Here's how the part is built. I have some questions about the finished solid (model axes, mm). Face numbers are marked on the shaded views. A direction names the side the tool comes from. Coordinates: 2 decimals unless noted, no trailing zeros. Write each loop counter-clockwise with the first axis right and the second up, starting at its lowest first coordinate (ties: lowest second). Pieces come first, ordered by that corner, then holes. Notation, with made-up numbers: (23.5, -39.75) -> (74.5, -39.75) arc R24 cw to (74.5, -8.75) -> close; hole circle Ø8 at (-9.75, -10.75). An arc over 180 degrees is marked (long way). Put each result on its own line as item: value. Start each with the question number.
Item 1: I want a section at A-A, the plane x = 35. List the corners of the cut face in (y, z) for me.
Item 2: I want a section at C-C, the plane x = 71.5. List the corners of the cut face in (y, z) for me, then the cut area to 3 significant figures.
Item 3: I need wall thicknesses on line 1 (Z direction, x = -147.5, y = 5.25); line 2 (Y direction, x = -29.5, z = -18.75); line 3 (Y direction, x = 100, z = -0.65). Which ranges of each line are inside material? Lowest first, please. Write a range as [from, to].
Item 4: If we mould it in two halves opening along Z, with no side actions, what happens to the marked faces 3, 4, 5 and 6? For each: released by +Z, released by -Z, zero draft, split by the parting line, or undercut.
Item 5: On a 3-axis mill with a long thin cutter (end or side, diameter ignored), from which of +Z, -Z, +X, -X, +Y, -Y can I reach the whole of each face in a straight line? I mean the marked faces 1 and 2. Say none if no direction works.
Item 6: I want a section at B-B, the plane z = -14.75. List the corners of the cut face in (x, y) for me, then the cut area to 3 significant figures.
from build123d import *

# Parameters (mm, degrees)
EXTRUDE_1_DEPTH     = 165
SKETCH_2_R          = 4.5
SKETCH_2_R_2        = 2
CUT_EXTRUDE_1_DEPTH = 171.367250374


with BuildPart() as part:
    # 草图1 → 凸台-拉伸1 (new, symmetric)
    with BuildSketch(Plane(origin=(0, 0, 0), x_dir=(0, 0, -1), z_dir=(1, 0, 0))):
        with BuildLine():
            Line((4, 0), (26, 0))
            ThreePointArc((26, 0), (28.828427125, 1.171572875), (30, 4))
            Line((30, 4), (30, 26))
            ThreePointArc((30, 26), (28.828427125, 28.828427125), (26, 30))
            Line((26, 30), (4, 30))
            ThreePointArc((4, 30), (1.171572875, 28.828427125), (0, 26))
            Line((0, 26), (0, 4))
            ThreePointArc((0, 4), (1.171572875, 1.171572875), (4, 0))
        make_face()
        with BuildLine():
            Line((4, 2), (26, 2))
            ThreePointArc((26, 2), (27.414213562, 2.585786438), (28, 4))
            Line((28, 4), (28, 26))
            ThreePointArc((28, 26), (27.414213562, 27.414213562), (26, 28))
            Line((26, 28), (4, 28))
            ThreePointArc((4, 28), (2.585786438, 27.414213562), (2, 26))
            Line((2, 26), (2, 4))
            ThreePointArc((2, 4), (2.585786438, 2.585786438), (4, 2))
        make_face(mode=Mode.SUBTRACT)
    extrude(amount=EXTRUDE_1_DEPTH, both=True)

    # 草图2 → 切除-拉伸1 (cut, through all)
    with BuildSketch(Plane.XY):
        with Locations((-35, 15)):
            Circle(SKETCH_2_R)
        with Locations((35, 15)):
            Circle(SKETCH_2_R)
        with Locations((-115, 15)):
            Circle(SKETCH_2_R_2)
        with Locations((115, 15)):
            Circle(SKETCH_2_R_2)
        with Locations((-100, 15)):
            Circle(SKETCH_2_R_2)
        with Locations((-90, 15)):
            Circle(SKETCH_2_R_2)
        with Locations((90, 15)):
            Circle(SKETCH_2_R_2)
        with Locations((100, 15)):
            Circle(SKETCH_2_R_2)
    extrude(amount=-CUT_EXTRUDE_1_DEPTH, mode=Mode.SUBTRACT)


solid = part.part
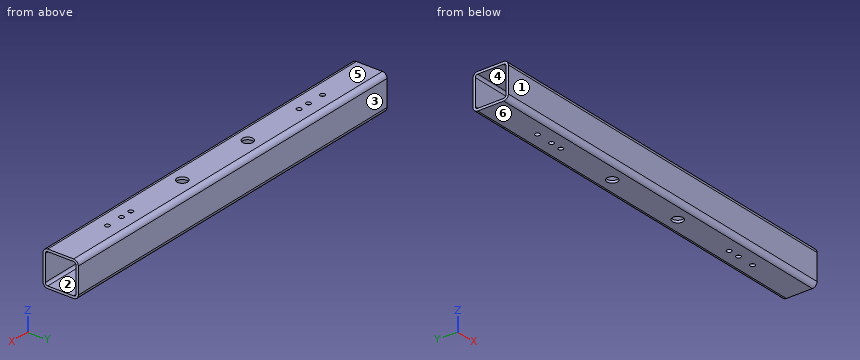
Calculated:
1. outline: (0, -26) arc R4 ccw to (4, -30) -> (10.5, -30) -> (10.5, -28) -> (4, -28) arc R2 cw to (2, -26) -> (2, -4) arc R2 cw to (4, -2) -> (10.5, -2) -> (10.5, 0) -> (4, 0) arc R4 ccw to (0, -4) -> close; (19.5, -30) -> (26, -30) arc R4 ccw to (30, -26) -> (30, -4) arc R4 ccw to (26, 0) -> (19.5, 0) -> (19.5, -2) -> (26, -2) arc R2 cw to (28, -4) -> (28, -26) arc R2 cw to (26, -28) -> (19.5, -28) -> close
2. outline: (0, -26) arc R4 ccw to (4, -30) -> (26, -30) arc R4 ccw to (30, -26) -> (30, -4) arc R4 ccw to (26, 0) -> (4, 0) arc R4 ccw to (0, -4) -> close; hole (2, -26) arc R2 ccw to (4, -28) -> (26, -28) arc R2 ccw to (28, -26) -> (28, -4) arc R2 ccw to (26, -2) -> (4, -2) arc R2 ccw to (2, -4) -> close
2. area: 214 mm2
3. line 1: z = [-30, -28], [-2, 0]
3. line 2: y = [0, 2], [28, 30]
3. line 3: y = [1.81, 13], [17, 28.19]
4. face 3: zero draft
4. face 4: undercut
4. face 5: released by +Z
4. face 6: released by -Z
5. face 1: +Z, -Z, +X, -X, -Y
5. face 2: +X, -X
6. outline: (-165, 0) -> (165, 0) -> (165, 2) -> (-165, 2) -> close; (-165, 28) -> (165, 28) -> (165, 30) -> (-165, 30) -> close
6. area: 1,320 mm2
